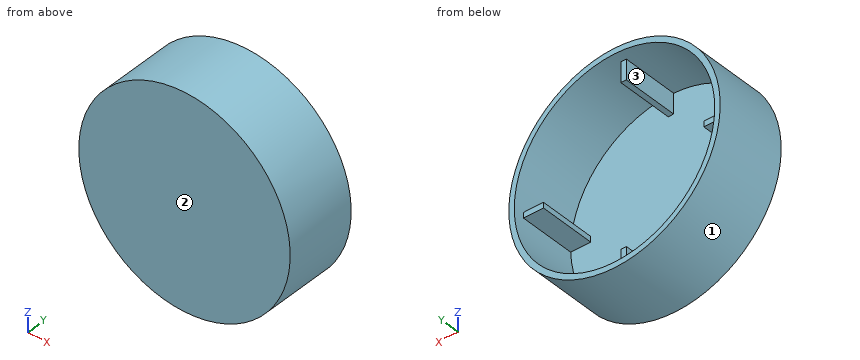
```python
from build123d import *

# Parameters (mm, degrees)
SKETCH1_R           = 29
BOSS_EXTRUDE1_DEPTH = 20
SHELL1_T            = -1.5
SKETCH2_W           = 1.5
SKETCH2_H           = 6.087803818
SKETCH2_W_2         = 6.087803818
SKETCH2_H_2         = 1.5
BOSS_EXTRUDE2_DEPTH = 15.5


with BuildPart() as part:
    # Sketch1 → Boss-Extrude1 (new body)
    with BuildSketch(Plane(origin=(0, 0, 0), x_dir=(1, 0, 0), z_dir=(0, 1, 0))):
        with Locations(Location((0, 0, 0), (0, 0, 270))):
            Circle(SKETCH1_R)
    extrude(amount=BOSS_EXTRUDE1_DEPTH)

    # Shell1
    shell1_openings = [part.faces().sort_by_distance(p)[0] for p in [
        (0, 20, 0),
    ]]
    offset(amount=SHELL1_T, openings=shell1_openings, kind=Kind.INTERSECTION)

    # Sketch2 → Boss-Extrude2 (add)
    with BuildSketch(Plane(origin=(0, 1.5, 0), x_dir=(1, 0, 0), z_dir=(0, 1, 0))):
        with Locations((0, 25.043901909)):
            Rectangle(SKETCH2_W, SKETCH2_H)
        with Locations((25.043901909, 0)):
            Rectangle(SKETCH2_W_2, SKETCH2_H_2)
        with Locations((0, -25.043901909)):
            Rectangle(SKETCH2_W, SKETCH2_H)
        with Locations((-25.043901909, 0)):
            Rectangle(SKETCH2_W_2, SKETCH2_H_2)
    extrude(amount=BOSS_EXTRUDE2_DEPTH)


solid = part.part
```
Work out the finished part from the listing and answer in its coordinate system (mm). Face numbers are marked on the shaded views. Round coordinates to 2 decimals unless told otherwise and drop trailing zeros. Write each loop counter-clockwise with the first axis right and the second up, starting at its lowest first coordinate (ties: lowest second). Pieces come first, ordered by that corner, then holes.
1) A cutting plane is placed at B-B on z = 0. Determine the outline of the cut face in (x, y).
2) Determine the mould class of the marked faces 1, 2 and 3 for opening direction X: pulls with the +X half, pulls with the -X half, needs draft (parallel to the pull), parting line crosses it, or undercut.
3) A cutting plane is placed at C-C on x = 0. Determine the outline of the cut face in (y, z).
4) A cutting plane is placed at A-A on y = 2.5. Determine the outline of the cut face in (x, z).
5) A cutting plane is placed at D-D on x = 20. Determine the outline of the cut face in (y, z), and give its area (3 significant figures).
6) Consider probe 1 along Z at (x, y) = (25, 14.5); probe 2 along X at (y, z) = (9.25, 0); probe 3 along Y at (x, z) = (-18, 20). Determine where each line is inside the solid, lowest interval first.
7) Flat-ended cylindrical pins translate along their axes: P1, Ø12, axis at y = 4.5, z = -23, coming from the -X side; P2, Ø0.8, axis at x = 26, z = 0, coming from the +Y side; P3, Ø16.5, axis at x = -5, z = 4, coming from the +Y side. Find the tip coordinate at first contact, or state that the pin passes through.
Entries:
1. outline: (-29, 0) - (29, 0) - (29, 20) - (27.5, 20) - (27.5, 17) - (22, 17) - (22, 1.5) - (-22, 1.5) - (-22, 17) - (-27.5, 17) - (-27.5, 20) - (-29, 20) - close
2. face 1: parting line crosses it
2. face 2: needs draft
2. face 3: undercut
3. outline: (0, -29) - (20, -29) - (20, -27.5) - (17, -27.5) - (17, -22) - (1.5, -22) - (1.5, 22) - (17, 22) - (17, 27.5) - (20, 27.5) - (20, 29) - (0, 29) - close
4. outline: circle Ø58 at (0, 0); hole (-27.49, -0.75) arc R27.5 ccw to (-0.75, -27.49) - (-0.75, -22) - (0.75, -22) - (0.75, -27.49) arc R27.5 ccw to (27.49, -0.75) - (22, -0.75) - (22, 0.75) - (27.49, 0.75) arc R27.5 ccw to (0.75, 27.49) - (0.75, 22) - (-0.75, 22) - (-0.75, 27.49) arc R27.5 ccw to (-27.49, 0.75) - (-22, 0.75) - (-22, -0.75) - close
5. outline: (0, -21) - (20, -21) - (20, -18.87) - (1.5, -18.87) - (1.5, 18.87) - (20, 18.87) - (20, 21) - (0, 21) - close
5. area: 142 mm2
6. probe 1: z = -14.7 to -11.46, -0.75 to 0.75, 11.46 to 14.7
6. probe 2: x = -29 to -22, 22 to 29
6. probe 3: y = 0 to 1.5
7. P1: stops at x = -23.49
7. P2: stops at y = 17
7. P3: stops at y = 1.5
